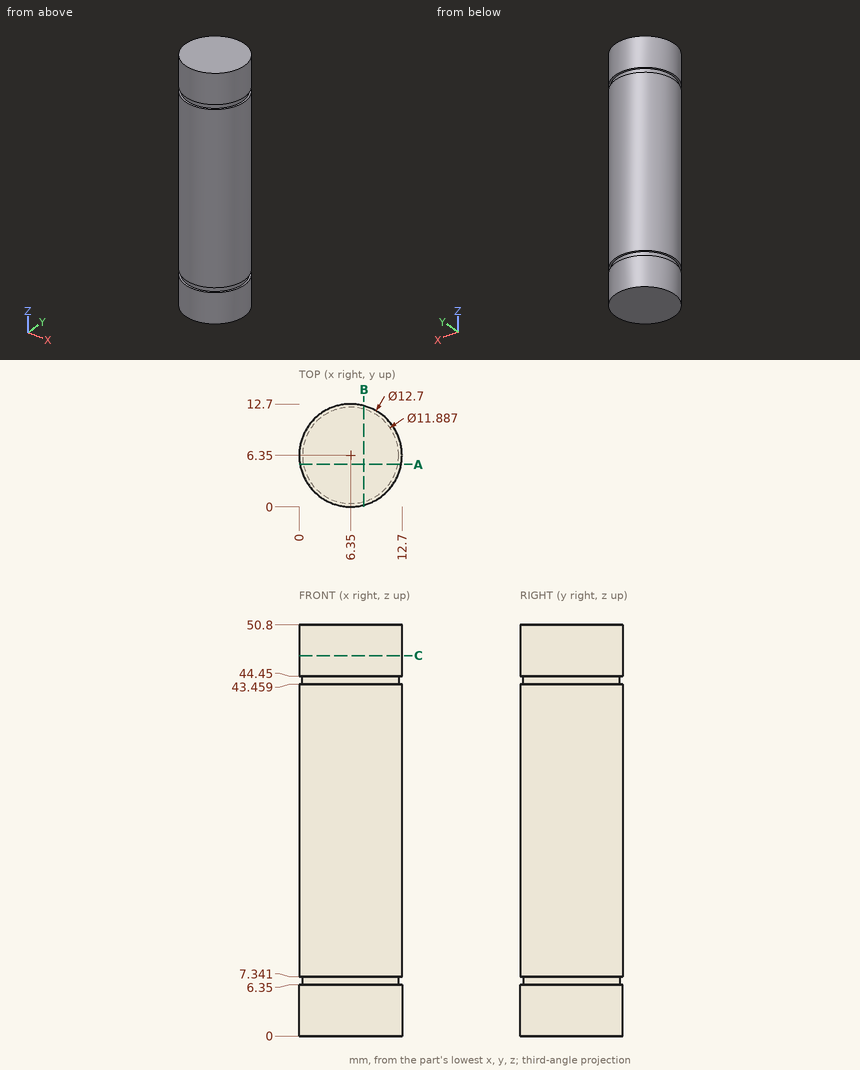
Design review of the part shown in the three views and the two pictorial views. Dimensions are in mm from the part's minimum x, y and z. Round coordinates to 2 decimals unless told otherwise and drop trailing zeros. Write each loop counter-clockwise with the first axis right and the second up, starting at its lowest first coordinate (ties: lowest second). Pieces come first, ordered by that corner, then holes.
Item 1: We need section B-B on x = 8. Write out the cut boundary in (y, z).
Item 2: Clearance check with a flat-ended pin moving along its axis: pin 1 Ø1 at (y, z) = (4, 39) entering from -X (1 decimal). State where the tip first meets the part, or that it passes through.
Item 3: We need section A-A on y = 5.25. Write out the cut boundary in (x, z).
Item 4: We need section C-C on z = 47. Write out the cut boundary in (x, y).
Item 5: For probe 1 along Z at (x, y) = (2, 10.5); probe 2 along X at (y, z) = (6.25, 45); probe 3 along Y at (x, z) = (5.25, 3.5) (1 decimal), list the stretches that pass through material, from the lowest coordinate up.
Returned:
1. outline: (0.22, 0) - (12.48, 0) - (12.48, 6.35) - (12.06, 6.35) - (12.06, 7.34) - (12.48, 7.34) - (12.48, 43.46) - (12.06, 43.46) - (12.06, 44.45) - (12.48, 44.45) - (12.48, 50.8) - (0.22, 50.8) - (0.22, 44.45) - (0.64, 44.45) - (0.64, 43.46) - (0.22, 43.46) - (0.22, 7.34) - (0.64, 7.34) - (0.64, 6.35) - (0.22, 6.35) - close
2. pin 1: stops at x = 0.3
3. outline: (0.1, 0) - (12.6, 0) - (12.6, 6.35) - (12.19, 6.35) - (12.19, 7.34) - (12.6, 7.34) - (12.6, 43.46) - (12.19, 43.46) - (12.19, 44.45) - (12.6, 44.45) - (12.6, 50.8) - (0.1, 50.8) - (0.1, 44.45) - (0.51, 44.45) - (0.51, 43.46) - (0.1, 43.46) - (0.1, 7.34) - (0.51, 7.34) - (0.51, 6.35) - (0.1, 6.35) - close
4. outline: circle Ø12.7 at (6.35, 6.35)
5. probe 1: z = 0 to 6.35, 7.34 to 43.46, 44.45 to 50.8
5. probe 2: x = 0 to 12.7
5. probe 3: y = 0.1 to 12.6
